```python
from build123d import *

# Parameters (mm, degrees)
F2_R     = 20
F3_DEPTH = 10.001


with BuildPart() as f1:
    # F0 (on Right) → F1 (revolve)
    with BuildSketch(Plane.YZ):
        Polygon((25, 5), (0, 5), (0, -5), (25, -5), (25, -3.5), (23.5, -3.5), (23.5, 3.5), (25, 3.5), align=None)
    revolve(axis=Axis((0, 0, 0), (0, 0, -1)))

    # F2 (on face) → F3 (cut, through all)
    with BuildSketch(Plane.XY.offset(5)):
        Circle(F2_R)
    extrude(amount=-F3_DEPTH, mode=Mode.SUBTRACT)


solid = f1.part
```
Read the model definition and answer for the solid it produces. Units are mm, in the model's axes. A direction names the side the tool comes from. Coordinates: 2 decimals unless noted, no trailing zeros. Write each loop counter-clockwise with the first axis right and the second up, starting at its lowest first coordinate (ties: lowest second). Pieces come first, ordered by that corner, then holes. Notation, with made-up numbers: (25.5, 9) -> (78.5, 9) arc R26 cw to (78.5, 34) -> close; hole circle Ø9 at (4, 25). An arc over 180 degrees is marked (long way). Answer as a JSON object with one key per item and string values.
Q1. A tool of negligible diameter and unlimited length cuts with its end or side. For faces 4 (the flat face through (17, 11, -5)), 5 (the flat face through (-17, -17, -3.5)), from which of +Z, -Z, +X, -X, +Y, -Y can it reach the whole face along a straight path? Write none if from no direction.
The answers:
{"face 4": "-Z, +X, -X, +Y, -Y", "face 5": "none"}
Q2. Consider line 1 (X direction, y = 0.5, z = -0.25); line 2 (X direction, y = 4, z = 2.25); line 3 (Y direction, x = 3, z = 1.5). Determine where each line is inside the solid, lowest interval first. Write a range as [from, to].
The answers:
{"line 1": "x = [-23.49, -19.99], [19.99, 23.49]", "line 2": "x = [-23.16, -19.6], [19.6, 23.16]", "line 3": "y = [-23.31, -19.77], [19.77, 23.31]"}
Q3. The part is cut by section A-A on y = 0. Give the vertices of the cut face in (x, z).
The answers:
{"outline": "(-25, -5) -> (-20, -5) -> (-20, 5) -> (-25, 5) -> (-25, 3.5) -> (-23.5, 3.5) -> (-23.5, -3.5) -> (-25, -3.5) -> close; (20, -5) -> (25, -5) -> (25, -3.5) -> (23.5, -3.5) -> (23.5, 3.5) -> (25, 3.5) -> (25, 5) -> (20, 5) -> close"}
Q4. The part is cut by section D-D on x = 21. Give the vertices of the cut face in (y, z).
The answers:
{"outline": "(-13.56, -5) -> (13.56, -5) -> (13.56, -3.5) -> (10.55, -3.5) -> (10.55, 3.5) -> (13.56, 3.5) -> (13.56, 5) -> (-13.56, 5) -> (-13.56, 3.5) -> (-10.55, 3.5) -> (-10.55, -3.5) -> (-13.56, -3.5) -> close"}
Q5. The part is cut by section C-C on y = 22.5. Give the vertices of the cut face in (x, z), then the cut area to 3 significant figures.
The answers:
{"outline": "(-10.9, -5) -> (10.9, -5) -> (10.9, -3.5) -> (6.78, -3.5) -> (6.78, 3.5) -> (10.9, 3.5) -> (10.9, 5) -> (-10.9, 5) -> (-10.9, 3.5) -> (-6.78, 3.5) -> (-6.78, -3.5) -> (-10.9, -3.5) -> close", "area": "160 mm2"}
Q6. Flat-ended cylindrical pins translate along their axes: pin 1 Ø2 at (x, z) = (14.5, 1.5) entering from -Y; pin 2 Ø4 at (y, z) = (18.5, 2.5) entering from -X; pin 3 Ø12 at (x, y) = (-9.5, -6) entering from -Z; pin 4 Ø3 at (x, z) = (9.5, -1.5) entering from +Y. Find the tip coordinate at first contact, or state that the pin passes through.
The answers:
{"pin 1": "stops at y = -19.24", "pin 2": "stops at x = -18.54", "pin 3": "passes through", "pin 4": "stops at y = 22.1"}
Q7. Determine the mould class of faces 1 (the cylindrical face through (-4.336, -19.524, 0.07)), 2 (the cylindrical face through (7.1, 22.4, 0)), 3 (the flat face through (17, -11, 5)) for opening direction Z: pulls with the +Z half, pulls with the -Z half, needs draft (parallel to the pull), parting line crosses it, or undercut.
The answers:
{"face 1": "needs draft", "face 2": "undercut", "face 3": "pulls with the +Z half"}
